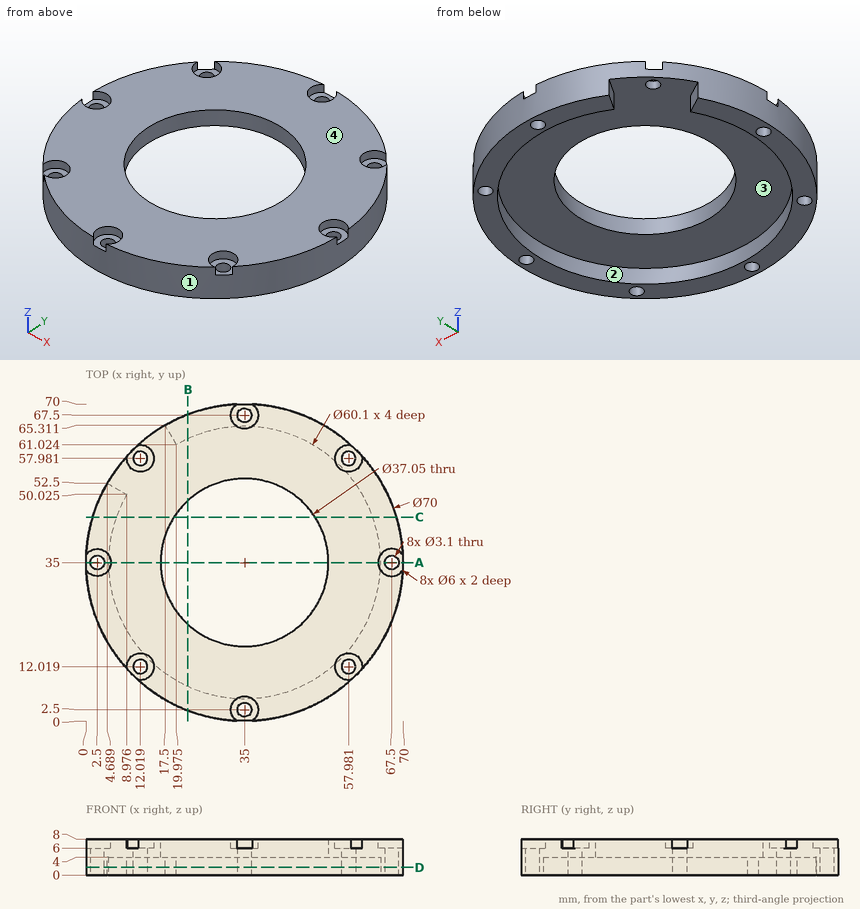
Job drawing, mm, ordinate dimensions from the low corner. One solid piece. Coordinates: 2 decimals unless noted, no trailing zeros. Order: outer loops, then holes, each group sorted by start corner. A loop starts at its lowest first (then second) coordinate and runs counter-clockwise, first axis right, second up. Notation, with made-up numbers: (30, 32) -> (63, 32) arc R32 cw to (63, 70) -> close; hole circle Ø1 at (62.5, 6.5). An arc over 180 degrees is marked (long way). Return JSON: item names as keys, results as strings. Group by question number.
Item 1: Saw through at A-A on y = 35. Write the cut outline in (x, z) (3 decimals), then the cut area to 3 significant figures.
Item 2: Wall check: line 1 along Y through (x, z) = (35, 5.35) (3 decimals); line 2 along Y through (x, z) = (35, 1.2); line 3 along Z through (x, y) = (6.5, 43). Give the ranges that are in metal, low to high. Write a range as [from, to].
Item 3: Saw through at D-D on z = 1.75. Write the cut outline in (x, y) (3 decimals).
Item 4: Flat gauge pins, fed straight in: P1, Ø2.5, axis at x = 35, y = 2.5, coming from the -Z side; P2, Ø4, axis at x = 53.5, z = 2, coming from the -Y side; P3, Ø5.5, axis at x = 35, y = 67.5, coming from the +Z side; P4, Ø1, axis at y = 47, z = 5, coming from the -X side. Where does each tip first touch, or does it go through?
Item 5: Saw through at B-B on x = 22.5. Write the cut outline in (y, z), then the cut area to 3 significant figures.
Item 6: Pull direction X, two halves, no side cores. Call the marked faces 1, 2, 3 and 4: pulls with the +X half, pulls with the -X half, needs draft (parallel to the pull), parting line crosses it, or undercut.
Item 7: Saw through at C-C on y = 45. Write the cut outline in (x, z).
Values found:
{
 "1": {"outline": "(0, 0) -> (0.95, 0) -> (0.95, 6) -> (0, 6) -> close; (4.05, 0) -> (4.95, 0) -> (4.95, 4) -> (16.475, 4) -> (16.475, 8) -> (5.5, 8) -> (5.5, 6) -> (4.05, 6) -> close; (53.525, 4) -> (65.05, 4) -> (65.05, 0) -> (65.95, 0) -> (65.95, 6) -> (64.5, 6) -> (64.5, 8) -> (53.525, 8) -> close; (69.05, 0) -> (70, 0) -> (70, 6) -> (69.05, 6) -> close", "area": "112 mm2"},
 "2": {"line 1": "y = [0, 0.95], [4.05, 16.475], [53.525, 65.95], [69.05, 70]", "line 2": "y = [0, 0.95], [4.05, 4.95], [65.05, 65.95], [69.05, 70]", "line 3": "z = [4, 8]"},
 "3": {"outline": "(4.689, 52.5) arc R35 ccw (long way) to (17.5, 65.311) -> (19.975, 61.024) arc R30.05 cw (long way) to (8.976, 50.025) -> close; hole circle Ø3.1 at (2.5, 35); hole circle Ø3.1 at (12.019, 12.019); hole circle Ø3.1 at (35, 2.5); hole circle Ø3.1 at (35, 67.5); hole circle Ø3.1 at (57.981, 12.019); hole circle Ø3.1 at (57.981, 57.981); hole circle Ø3.1 at (67.5, 35)"},
 "4": {"P1": "passes through", "P2": "stops at y = 4.13", "P3": "stops at z = 6", "P4": "stops at x = 1.94"},
 "5": {"outline": "(2.31, 0) -> (7.67, 0) -> (7.67, 4) -> (21.33, 4) -> (21.33, 8) -> (2.31, 8) -> close; (48.67, 4) -> (62.33, 4) -> (62.33, 0) -> (67.69, 0) -> (67.69, 8) -> (48.67, 8) -> close", "area": "195 mm2"},
 "6": {"face 1": "parting line crosses it", "face 2": "undercut", "face 3": "undercut", "face 4": "needs draft"},
 "7": {"outline": "(1.46, 0) -> (6.66, 0) -> (6.66, 4) -> (19.41, 4) -> (19.41, 8) -> (1.46, 8) -> close; (50.59, 4) -> (63.34, 4) -> (63.34, 0) -> (68.54, 0) -> (68.54, 8) -> (50.59, 8) -> close"}
}
